from build123d import *

# Parameters (mm, degrees)
F1_DEPTH      = 15
F3_DEPTH      = 15
F3_DEPTH_BACK = 7
F6_DEPTH      = 20
F7_DEPTH      = 20


with BuildPart() as f1:
    # F0 (on Top) → F1 (new body)
    with BuildSketch(Plane.XY):
        with BuildLine():
            Line((0, 0), (7, 0))
            ThreePointArc((7, 0), (4.9497474683, 4.9497474683), (0, 7))
            Line((0, 7), (0, 0))
        make_face()
    extrude(amount=F1_DEPTH)


with BuildPart() as f3:
    # F2 (on face) → F3 (new body, two sides)
    with BuildSketch(Plane.XZ) as f3_sk:
        with BuildLine():
            ThreePointArc((7, 8), (4.9497474683, 12.9497474683), (0, 15))
            Line((0, 15), (0, 8))
            Line((0, 8), (7, 8))
        make_face()
    extrude(amount=F3_DEPTH)
    extrude(f3_sk.sketch, amount=-F3_DEPTH_BACK)

    # F4: intersect F1
    add(f1.part, mode=Mode.INTERSECT)

    # F6 (add): a face of the model
    f6_faces = [f3.faces().sort_by_distance(p)[0] for p in [
        (2.970892271, 0, 10.970892271),
    ]]
    extrude(f6_faces, amount=F6_DEPTH)

    # F5 (on face) → F7 (join)
    with BuildSketch(Plane(origin=(0, 0, 8), x_dir=(1, 0, 0), z_dir=(0, 0, -1))):
        with BuildLine():
            ThreePointArc((0, -7), (4.9497474683, -4.9497474683), (7, 0))
            Line((7, 0), (0, 0))
            Line((0, 0), (0, -7))
        make_face()
    extrude(amount=F7_DEPTH)


solid = f3.part
Geometry check sheet. Reference: the model listing, model coordinates, mm. A direction names the side the tool comes from. Give positions to 0.01 mm unless a question says otherwise; leave off trailing zeros. Loops run counter-clockwise (first coordinate to the right, second up) from the corner with the lowest first, then second, coordinate; pieces in that order, holes last.
(1) Section check A-A on y = -13. Record the cut outline in (x, z), then the cut area to 3 significant figures.
From the geometry:
outline: (0, 8) - (7, 8) arc R7 ccw to (0, 15) - close
area: 38.5 mm2
(2) Depth check by flat-ended pin: pin 1 Ø4 at (x, z) = (5.5, 11) entering from +Y; pin 2 Ø1 at (x, z) = (4.5, 1) entering from -Y; pin 3 Ø2 at (x, y) = (2.5, -10.5) entering from -Z. Enter the tip coordinate at first touch or a pass-through.
From the geometry:
pin 1: stops at y = 6.06
pin 2: stops at y = 0
pin 3: stops at z = 8
(3) Thickness scan on L1, parallel to Z at x = 2, y = -9.5; L2, parallel to Y at x = 1.5, z = 10.25; L3, parallel to Z at x = 5.75, y = -1. Record the ranges inside material, lowest first.
From the geometry:
L1: z = 8 to 14.71
L2: y = -20 to 6.84
L3: z = 8 to 11.99
(4) Set-up check for faces 1 (the flat face through (4, 0, -2)), 2 (the cylindrical face through (5, -6.3, 12.9)): record each of +Z, -Z, +X, -X, +Y, -Y from which the full face is reachable in a straight line by a thin tool's end or side.
From the geometry:
face 1: -Z, +X, -X, -Y
face 2: +Z, +X, +Y, -Y
(5) Release check for a two-part mould opening along X. For faces 3 (the cylindrical face through (4.9, 5, 1.7)), 4 (the flat face through (3, -10, 8)), 5 (the flat face through (0, 2, 8)) record: released by +X, released by -X, zero draft, split by the parting line, or undercut.
From the geometry:
face 3: released by +X
face 4: zero draft
face 5: released by -X
(6) Section check C-C on x = 4. Record the cut outline in (y, z), then the cut area to 3 significant figures.
From the geometry:
outline: (-20, 8) - (0, 8) - (0, -12) - (5.74, -12) - (5.74, 13.74) - (-20, 13.74) - close
area: 263 mm2
(7) Section check B-B on z = -2.75. Record the cut outline in (x, y).
From the geometry:
outline: (0, 0) - (7, 0) arc R7 ccw to (0, 7) - close
(8) Section check D-D on x = 0.5. Record the cut outline in (y, z).
From the geometry:
outline: (-20, 8) - (0, 8) - (0, -12) - (6.98, -12) - (6.98, 14.98) - (-20, 14.98) - close
